Input: dimensioned drawing with shaded views. Units: mm. Origin: part minimum x, y, z. Round coordinates to 2 decimals unless told otherwise and drop trailing zeros. Loops run counter-clockwise (first coordinate to the right, second up) from the corner with the lowest first, then second, coordinate; pieces in that order, holes last. Notation, with made-up numbers: M 67.25,-32.75 L 109.25,-32.75 A18 ccw 109.25,-15.75 Z; hole C 40.25,-4.75 d9. An arc over 180 degrees is marked long. Write each question's results on one line, items separated by ' | '. Start each with the question number.
1. Section A-A on z = 72. Output: boundary loops of the cut face in (x, y), and give its area (3 significant figures).
2. Ray query, line 1 (X direction, y = 2.85, z = 104.5); line 2 (Z direction, x = 180, y = 5.5); line 3 (X direction, y = 4.2, z = 107). Return the intervals inside material, ascending.
3. Section D-D on x = 86.5. Output: boundary loops of the cut face in (y, z).
4. Section C-C on x = 388. Output: boundary loops of the cut face in (y, z), and give its area (3 significant figures).
5. Contact query for a flat-ended pin moving along its axis: pin 1 Ø3 at (x, y) = (316.5, 2) entering from +Z. Output: stop coordinate, or through.
6. Section B-B on y = 4.75. Output: boundary loops of the cut face in (x, z).
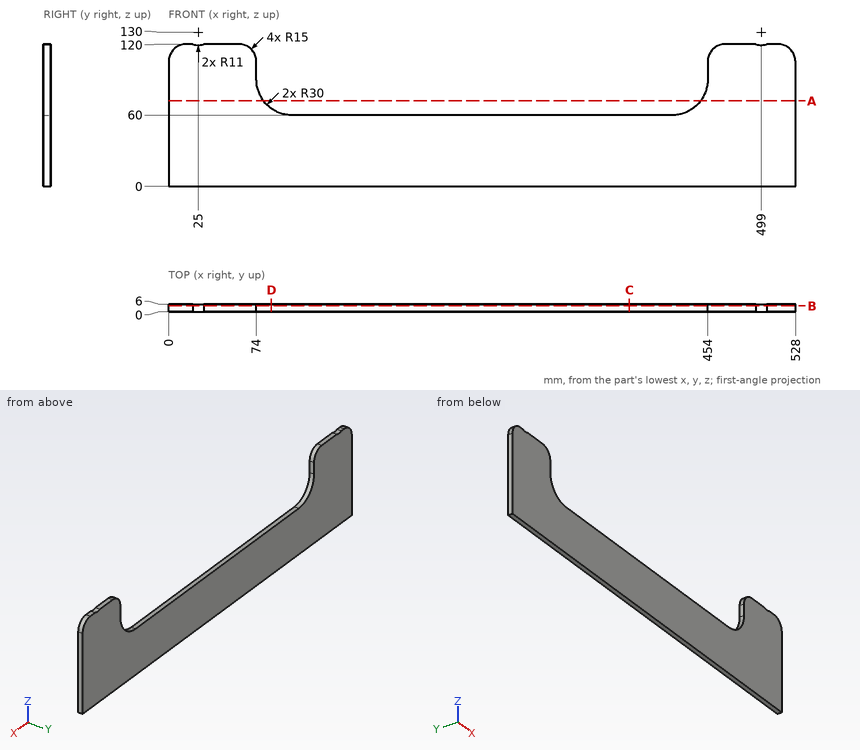
Taken from the geometry:
1) outline: M 0,0 L 80,0 L 80,6 L 0,6 Z; M 448,0 L 528,0 L 528,6 L 448,6 Z | area: 960 mm^2
2) line 1: 0 to 74, 454 to 528 | line 2: 0 to 60 | line 3: 0.13 to 73.87, 454.13 to 527.87
3) outline: M 0,0 L 6,0 L 6,65.63 L 0,65.63 Z
4) outline: M 0,0 L 6,0 L 6,60 L 0,60 Z | area: 360 mm^2
5) pin 1: z = 60
6) outline: M 0,0 L 528,0 L 528,105 A15 ccw 513,120 L 503.58,120 A11 cw 494.42,120 L 469,120 A15 ccw 454,105 L 454,90 A30 cw 424,60 L 104,60 A30 cw 74,90 L 74,105 A15 ccw 59,120 L 29.58,120 A11 cw 20.42,120 L 15,120 A15 ccw 0,105 Z
